```python
from build123d import *

# Parameters (mm, degrees)
SKETCH2_R             = 2.5
BOSS_EXTRUDE1_DEPTH   = 27
CHAMFER1_SIZE         = 0.1
CHAMFER1_SIZE2        = 0.173205081
CHAMFER1_PART_2_SIZE  = 0.1
CHAMFER1_PART_2_SIZE2 = 0.173205081
M3X0_5_TAPPED_HOLE1_D = 2.5


with BuildPart() as part:
    # Sketch2 → Boss-Extrude1 (new body)
    with BuildSketch(Plane(origin=(0, 0, 0), x_dir=(1, 0, 0), z_dir=(0, 1, 0))):
        Circle(SKETCH2_R)
    extrude(amount=BOSS_EXTRUDE1_DEPTH)

    # Chamfer1
    chamfer1_edges = [part.edges().sort_by_distance(p)[0] for p in [
        (-2.5, 0, 0),
    ]]
    chamfer1_side = [part.faces().sort_by_distance(p)[0] for p in [
        (0, 0, 0),
    ]]
    chamfer(chamfer1_edges, length=CHAMFER1_SIZE, length2=CHAMFER1_SIZE2, reference=chamfer1_side[0])

    # Chamfer1 part 2
    chamfer1_part_2_edges = [part.edges().sort_by_distance(p)[0] for p in [
        (-2.5, 27, 0),
    ]]
    chamfer1_part_2_side = [part.faces().sort_by_distance(p)[0] for p in [
        (-2.5, 13.5, 0),
    ]]
    chamfer(chamfer1_part_2_edges, length=CHAMFER1_PART_2_SIZE, length2=CHAMFER1_PART_2_SIZE2, reference=chamfer1_part_2_side[0])

    # M3x0.5 Tapped Hole1 (through all)
    with Locations(Plane(origin=(0, 27, 0), x_dir=(1, 0, 0), z_dir=(0, 1, 0))):
        with Locations((0, 0)):
            Hole(M3X0_5_TAPPED_HOLE1_D / 2)


solid = part.part
```
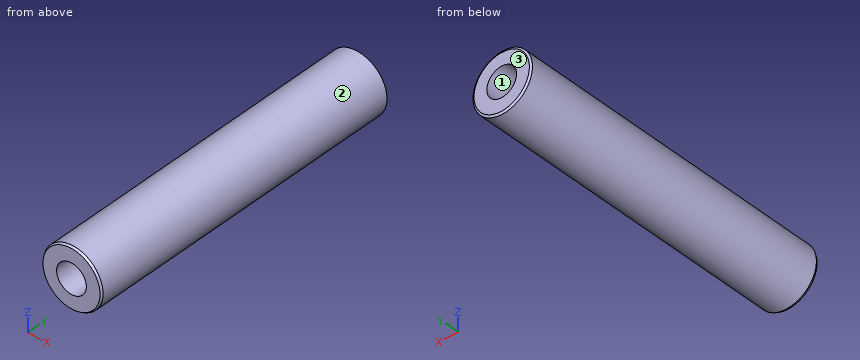
Geometry check sheet. Reference: the model listing, model coordinates, mm. Face numbers are marked on the shaded views. Coordinates: 2 decimals unless noted, no trailing zeros. Order: outer loops, then holes, each group sorted by start corner. A loop starts at its lowest first (then second) coordinate and runs counter-clockwise, first axis right, second up. Notation, with made-up numbers: M 15,-20 L 53,-20 A13 cw 53,-7 Z; hole C 83,2.25 d10. An arc over 180 degrees is marked long. Answer as a JSON object with one key per item and string values.
Q1. Cross-section at B-B on z = 0. Record the cut outline in (x, y).
Results are:
{"outline": "M -2.5,0.17 L -2.4,0 L -1.25,0 L -1.25,27 L -2.33,27 L -2.5,26.9 Z; M 1.25,0 L 2.4,0 L 2.5,0.17 L 2.5,26.9 L 2.33,27 L 1.25,27 Z"}
Q2. Cross-section at A-A on x = 0. Record the cut outline in (y, z), and give its area (3 significant figures).
Results are:
{"outline": "M 0,-2.4 L 0.17,-2.5 L 26.9,-2.5 L 27,-2.33 L 27,-1.25 L 0,-1.25 Z; M 0,1.25 L 27,1.25 L 27,2.33 L 26.9,2.5 L 0.17,2.5 L 0,2.4 Z", "area": "67.5 mm²"}
Q3. Release check for a two-part mould opening along Z. For the marked faces 1, 2 and 3 record: released by +Z, released by -Z, zero draft, split by the parting line, or undercut.
Results are:
{"face 1": "undercut", "face 2": "split by the parting line", "face 3": "zero draft"}
Q4. Scan lines: line 1 (Z direction, x = 0, y = 21.5); line 2 (X direction, y = 10.25, z = -1.1) (3 decimals); line 3 (X direction, y = 20.25, z = 0.8). Record each from-to range of solid material in increasing order.
Results are:
{"line 1": "z = -2.5 to -1.25, 1.25 to 2.5", "line 2": "x = -2.245 to -0.594, 0.594 to 2.245", "line 3": "x = -2.37 to -0.96, 0.96 to 2.37"}
Q5. Depth check by flat-ended pin: pin 1 Ø1.5 at (x, y) = (0.5, 15) entering from -Z. Enter the tip coordinate at first touch or a pass-through.
Results are:
{"pin 1": "stops at z = -2.5"}
Q6. Cross-section at C-C on y = 8.25. Record the cut outline in (x, z).
Results are:
{"outline": "C 0,0 d5; hole C 0,0 d2.5"}
